Part model, mm, in its own coordinate system. Face numbers are marked on the shaded views. A direction names the side the tool comes from. Coordinates: 2 decimals unless noted, no trailing zeros. Order: outer loops, then holes, each group sorted by start corner. A loop starts at its lowest first (then second) coordinate and runs counter-clockwise, first axis right, second up.
```python
from build123d import *

# Parameters (mm, degrees)
SKETCH_1_R          = 1.55
EXTRUDE_1_DEPTH     = 1
FILLET_1_R          = 0.6
EXTRUDE_2_DEPTH     = 2
SKETCH_3_R          = 0.6
CUT_EXTRUDE_1_DEPTH = 3
FILLET_2_R          = 0.5
FILLET_3_R          = 1


with BuildPart() as part:
    # 草图1 → 凸台-拉伸1 (new body, symmetric)
    with BuildSketch(Plane.XY):
        with BuildLine():
            Line((0, -3), (-15, -3))
            Line((-15, -3), (-15, 0))
            Line((-15, 0), (11.490666647, 9.641814145))
            Line((11.490666647, 9.641814145), (13.419029476, 7.343680816))
            Line((13.419029476, 7.343680816), (1.928362829, -2.298133329))
            ThreePointArc((1.928362829, -2.298133329), (1.02606043, -2.819077862), (0, -3))
        make_face()
        Circle(SKETCH_1_R, mode=Mode.SUBTRACT)
        with BuildLine():
            Line((-13.361770819, -1), (-3.364453737, 2.63872584))
            ThreePointArc((-3.364453737, 2.63872584), (-2.579616657, 2.419704921), (-2.533815922, 1.606168383))
            ThreePointArc((-2.533815922, 1.606168383), (-2.981013424, 0.336985115), (-2.828427125, -1))
            Line((-2.828427125, -1), (-13.361770819, -1))
        make_face(mode=Mode.SUBTRACT)
        with BuildLine():
            Line((10.878497896, 7.822736283), (2.809488491, 1.052033468))
            ThreePointArc((2.809488491, 1.052033468), (2.066978912, 2.174304068), (0.908590471, 2.859101844))
            ThreePointArc((0.908590471, 2.859101844), (0.420744663, 3.511747133), (0.881180814, 4.184010443))
            Line((0.881180814, 4.184010443), (10.878497896, 7.822736283))
        make_face(mode=Mode.SUBTRACT)
    extrude(amount=EXTRUDE_1_DEPTH, both=True)

    # 圆角1
    fillet_1_edges = [part.edges().sort_by_distance(p)[0] for p in [
        (-13.361770819, -1, 0),
        (-2.828427125, -1, 0),
        (10.878497896, 7.822736283, 0),
        (2.809488491, 1.052033468, 0),
    ]]
    fillet(fillet_1_edges, radius=FILLET_1_R)

    # 草图2 → 凸台-拉伸2 (add)
    with BuildSketch(Plane.XY.offset(1)):
        Polygon((-12, -3), (-10, -3), (-10, -5.5), (-5, -5.5), (-5, -3), (-3, -3), (-3, -7), (-12, -7), align=None)
        Polygon((11.120896146, 5.415317987), (13.692046585, 2.351140214), (6.797646597, -3.433948273), (4.226496158, -0.3697705), (5.758585045, 0.915804719), (7.365554069, -0.999306389), (11.195776284, 2.21463166), (9.58880726, 4.129742768), align=None)
    extrude(amount=-EXTRUDE_2_DEPTH)

    # 草图3 → 切除-拉伸1 (cut, through all)
    with BuildSketch(Plane.XY.offset(1)):
        with Locations((-5.6, -3)):
            Circle(SKETCH_3_R)
        with Locations((-5.6, -5.5)):
            Circle(SKETCH_3_R)
        with Locations((-9.4, -3)):
            Circle(SKETCH_3_R)
        with Locations((-9.4, -5.5)):
            Circle(SKETCH_3_R)
        with Locations((6.218211711, 1.301477285)):
            Circle(SKETCH_3_R)
        with Locations((7.825180735, -0.613633823)):
            Circle(SKETCH_3_R)
        with Locations((9.129180594, 3.744070202)):
            Circle(SKETCH_3_R)
        with Locations((10.736149619, 1.828959094)):
            Circle(SKETCH_3_R)
        with Locations((-12.6, -3)):
            Circle(SKETCH_3_R)
        with Locations((-2.4, -3)):
            Circle(SKETCH_3_R)
        with Locations((3.766869493, -0.755443066)):
            Circle(SKETCH_3_R)
        with Locations((11.580522812, 5.800990553)):
            Circle(SKETCH_3_R)
    extrude(amount=-CUT_EXTRUDE_1_DEPTH, mode=Mode.SUBTRACT)

    # 圆角2
    fillet_2_edges = [part.edges().sort_by_distance(p)[0] for p in [
        (13.692046585, 2.351140214, 0),
        (6.797646597, -3.433948273, 0),
        (-12, -7, 0),
        (-3, -7, 0),
    ]]
    fillet(fillet_2_edges, radius=FILLET_2_R)

    # 圆角3
    fillet_3_edges = [part.edges().sort_by_distance(p)[0] for p in [
        (-15, 0, 0),
        (11.490666647, 9.641814145, 0),
    ]]
    fillet(fillet_3_edges, radius=FILLET_3_R)


solid = part.part
```
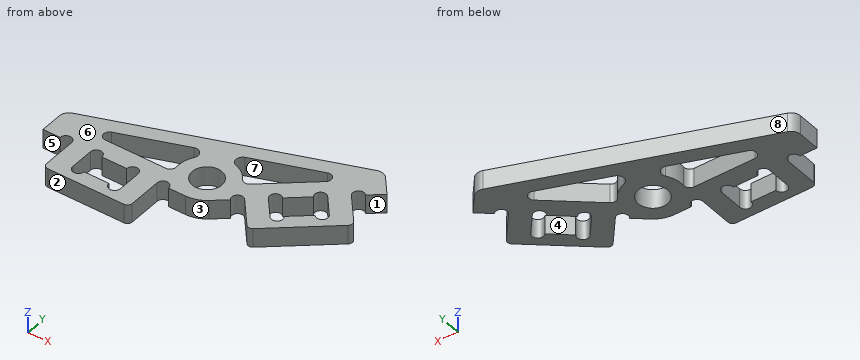
(1) Tool access for the marked faces 1, 2, 3 and 4: list every direction of +Z, -Z, +X, -X, +Y, -Y with a clear straight run to the whole face (end or side of a thin tool).
(2) Slice it at D-D, the plane x = -12.6. Give the cut face in (y, z), then the cut area to 3 significant figures.
(3) Slice it at A-A, the plane y = -5. Give the cut face in (x, z).
(4) Slice it at C-C, the plane z = -0.35. State how many separate pieces and enclosed holes the cut face has, then the cut area to 3 significant figures.
(5) Slice it at B-B, the plane x = -9.4. Give the cut face in (y, z), then the cut area to 3 significant figures.
(6) Probe line 1 (X direction, y = -6, z = 0.85); line 2 (X direction, y = -0.25, z = 0.3); line 3 (Y direction, x = -9, z = 0.45). List the from-to ranges inside material, lowest first.
(7) Pull direction Y, two halves, no side cores. Call the marked faces 5, 6, 7 and 8: +Y half, -Y half, draft (parallel to the pull), parting line (faces both ways), or undercut.
(8) Drop flat-ended pins along their axis: pin 1 (1 mm diameter, centred on x = -7, z = 0.5, fed in from +Y); pin 2 (0.6 mm diameter, centred on y = -3.5, z = -0.5, fed in from -X); pin 3 (1.9 mm diameter, centred on x = 0, y = 0, fed in from +Z); pin 4 (1 mm diameter, centred on x = -11, z = 0.5, fed in from +Y). Give the stop position or say it passes through.
Here are the results:
1. face 1: +Z, -Z, +X
1. face 2: +Z, -Z, +X, -X, -Y
1. face 3: +Z, -Z, -Y
1. face 4: +Z, -Z
2. outline: (-2.4, -1) - (0.87, -1) - (0.87, 1) - (-2.4, 1) - close
2. area: 6.55 mm2
3. outline: (-12, -1) - (-10, -1) - (-10, 1) - (-12, 1) - close; (-5, -1) - (-3, -1) - (-3, 1) - (-5, 1) - close
4. separate pieces: 1
4. enclosed holes: 5
4. area: 160 mm2
5. outline: (-7, -1) - (-6.1, -1) - (-6.1, 1) - (-7, 1) - close; (-2.4, -1) - (-1, -1) - (-1, 1) - (-2.4, 1) - close; (0.44, -1) - (2.04, -1) - (2.04, 1) - (0.44, 1) - close
5. area: 7.79 mm2
6. line 1: x = -12 to -9.73, -9.07 to -5.93, -5.27 to -3
6. line 2: x = -14.89 to -10.54, -2.99 to -1.53, 1.53 to 3.44, 4.09 to 6.74, 8.3 to 10.59
6. line 3: y = -7 to -5.95, -2.55 to -1, 0.59 to 2.18
7. face 5: -Y half
7. face 6: draft
7. face 7: undercut
7. face 8: +Y half
8. pin 1: stops at y = 3.09
8. pin 2: stops at x = -12
8. pin 3: passes through
8. pin 4: stops at y = 1.64
